Could you check a few things on this model? Use its own coordinates, in mm. A direction names the side the tool comes from. Coordinates: 2 decimals unless noted, no trailing zeros. Write each loop counter-clockwise with the first axis right and the second up, starting at its lowest first coordinate (ties: lowest second). Pieces come first, ordered by that corner, then holes.
Item 1: If I drill on probe 1 along Y at (x, z) = (-34, 4); probe 2 along Y at (x, z) = (-26.5, 8); probe 3 along Y at (x, z) = (-2, 2.5), over which ranges is the centre line in solid material (lowest first)?
Item 2: For P1, Ø6, axis at x = -31.5, y = 6, coming from the -Z side; P2, Ø1.5, axis at y = 7, z = 7, coming from the -X side; P3, Ø4, axis at y = -14, z = 7.5, coming from the -X side; P4, Ø3, axis at y = 19, z = 9, coming from the +X side, each with a flat end and sliding along its axis, tell me the tip position at first contact or that it passes through.
Item 3: I want a section at C-C on x = 41. Please give me the cut outline in (y, z), then the cut area to 3 significant figures.
Item 4: I want a section at A-A on x = 0. Please give me the cut outline in (y, z), then the cut area to 3 significant figures.
Item 5: Which directions (+Z, -Z, +X, -X, +Y, -Y) give clear straight access to the entire face, cutting with the end or side of a thin tool? Please do faces 4 (the flat face through (27, -34.127, 5)), 5 (the cylindrical face through (31.238, 9.837, 4.536)), 6 (the flat face through (-34.192, -30.183, 1.06)).
Item 6: Thinking about a two-plate mould opening in Y: for faces 1 (the cylindrical face through (-44.68, 36.27, 5.07)), 2 (the cylindrical face through (50.87, 42.69, 5.68)), 3 (the flat face through (34.667, -30.315, 7.357)), which applies, +Y half, -Y half, draft (parallel to the pull), parting line (faces both ways), or undercut?
from build123d import *

# Parameters (mm, degrees)
SKIZZE1_R                       = 32.75
AUFSATZ_LINEAR_AUSTRAGEN1_DEPTH = 10
AUFSATZ_LINEAR_START            = -0.8
SKIZZE2_R                       = 32.75
SKIZZE2_R_2                     = 30.25
AUFSATZ_LINEAR_AUSTRAGEN2_DEPTH = 0.8
SKIZZE5_R                       = 2.25
SCHNITT_LINEAR_AUSTRAGEN1_DEPTH = 10
VERRUNDUNG1_R                   = 50
VERRUNDUNG2_R                   = 6
VERRUNDUNG3_R                   = 4
AUFSATZ_LINEAR_AUSTRAGEN3_DEPTH = 8.306468


with BuildPart() as part:
    # Skizze1 → Aufsatz-Linear austragen1 (new body)
    with BuildSketch(Plane.XY):
        with BuildLine():
            Line((-13.635878322, -34.12660725), (-33.089645956, -34.12660725))
            Line((-33.089645956, -34.12660725), (-35.325135331, -26.12660725))
            Line((-35.325135331, -26.12660725), (-25.844978112, -26.12660725))
            ThreePointArc((-25.844978112, -26.12660725), (-36.75, 0), (-25.844978112, 26.12660725))
            Line((-25.844978112, 26.12660725), (-50.235580292, 27.232429468))
            Line((-50.235580292, 27.232429468), (-52.656417654, 35.895722216))
            Line((-52.656417654, 35.895722216), (-56.424186432, 49.379190555))
            Line((-56.424186432, 49.379190555), (-49.682452262, 51.263074944))
            Line((-49.682452262, 51.263074944), (-45.294995525, 35.561969729))
            Line((-45.294995525, 35.561969729), (-13.635878322, 34.12660725))
            ThreePointArc((-13.635878322, 34.12660725), (0, 36.75), (13.635878322, 34.12660725))
            Line((13.635878322, 34.12660725), (45.294995525, 35.561969729))
            Line((45.294995525, 35.561969729), (49.682452262, 51.263074944))
            Line((49.682452262, 51.263074944), (56.424186432, 49.379190555))
            Line((56.424186432, 49.379190555), (52.656417654, 35.895722216))
            Line((52.656417654, 35.895722216), (50.235580292, 27.232429468))
            Line((50.235580292, 27.232429468), (25.844978112, 26.12660725))
            ThreePointArc((25.844978112, 26.12660725), (36.75, 0), (25.844978112, -26.12660725))
            Line((25.844978112, -26.12660725), (35.325135331, -26.12660725))
            Line((35.325135331, -26.12660725), (33.089645956, -34.12660725))
            Line((33.089645956, -34.12660725), (13.635878322, -34.12660725))
            ThreePointArc((13.635878322, -34.12660725), (0, -36.75), (-13.635878322, -34.12660725))
        make_face()
        Circle(SKIZZE1_R, mode=Mode.SUBTRACT)
    extrude(amount=AUFSATZ_LINEAR_AUSTRAGEN1_DEPTH)

    # Skizze2 → Aufsatz-Linear austragen2 (add)
    with BuildSketch(Plane.XY.offset(10).offset(AUFSATZ_LINEAR_START)):
        Circle(SKIZZE2_R)
        Circle(SKIZZE2_R_2, mode=Mode.SUBTRACT)
    extrude(amount=AUFSATZ_LINEAR_AUSTRAGEN2_DEPTH)

    # Skizze5 → Schnitt-Linear austragen1 (cut)
    with BuildSketch(Plane(origin=(32.796772797, -9.164604643, 0), x_dir=(0, 0, 1), z_dir=(-0.9631048813334842, 0.2691263412444341, 0))):
        with Locations(Location((5, 56.94978804, 0), (0, 0, 270))):
            Circle(SKIZZE5_R)
    schnitt_linear_austragen1 = extrude(amount=-SCHNITT_LINEAR_AUSTRAGEN1_DEPTH, mode=Mode.SUBTRACT)

    # Spiegeln1: Schnitt-Linear austragen1 across plane
    add(schnitt_linear_austragen1.mirror(Plane(origin=(0, 0, 0), x_dir=(0, 0, 1), z_dir=(1, 0, 0))), mode=Mode.SUBTRACT)

    # Verrundung1
    verrundung1_edges = [part.edges().sort_by_distance(p)[0] for p in [
        (13.635878322, 34.12660725, 5),
        (13.635878322, -34.12660725, 5),
        (-13.635878322, -34.12660725, 5),
        (-13.635878322, 34.12660725, 5),
    ]]
    fillet(verrundung1_edges, radius=VERRUNDUNG1_R)

    # Verrundung2
    # the kernel refuses this fillet: 6 mm, written as the material it adds along each edge
    with BuildSketch(Plane(origin=(-25.844978112, -26.12660725, 0), x_dir=(-1, 0, 0), z_dir=(0, 0, 1))) as verrundung2_piece_1:
        with BuildLine():
            CenterArc((11.651069987, -5.593490659), VERRUNDUNG2_R, 111.211936516, 97.493506366)
            Line((6.388466745, -8.475331584), (6.283214681, -8.532968403))
            ThreePointArc((6.283214681, -8.532968403), (3.405977683, -4.078058883), (-0.084391765, -0.085311371))
            Line((-0.084391765, -0.085311371), (0, 0.12))
            ThreePointArc((0, 0.12), (4.74007861, 0.12), (9.436738964, 0.111869813))
            Line((9.436738964, 0.111869813), (9.48015722, 0))
        make_face()
    extrude(amount=10)
    with BuildSketch(Plane(origin=(25.844978112, -26.12660725, 0), x_dir=(1, 0, 0), z_dir=(0, 0, 1))) as verrundung2_piece_2:
        with BuildLine():
            CenterArc((11.651069987, 5.593490659), VERRUNDUNG2_R, 151.294557118, 97.493506366)
            Line((6.388466745, 8.475331584), (6.283214681, 8.532968403))
            ThreePointArc((6.283214681, 8.532968403), (3.405977683, 4.078058883), (-0.084391765, 0.085311371))
            Line((-0.084391765, 0.085311371), (0, -0.12))
            ThreePointArc((0, -0.12), (4.74007861, -0.12), (9.436738964, -0.111869813))
            Line((9.436738964, -0.111869813), (9.48015722, 0))
        make_face()
    extrude(amount=10)
    with BuildSketch(Plane(origin=(25.844978112, 26.12660725, 0), x_dir=(0.603126946859045, -0.7976452130944475, 0), z_dir=(0, 0, 1))) as verrundung2_piece_3:
        with BuildLine():
            CenterArc((11.361383868, 5.938413704), VERRUNDUNG2_R, 145.501722428, 116.281978681)
            Line((6.416524574, 9.336702474), (6.317627388, 9.40466825))
            Line((6.317627388, 9.40466825), (-0.098897186, 0.067965775))
            Line((-0.098897186, 0.067965775), (0.017149259, -0.118768274))
            ThreePointArc((0.017149259, -0.118768274), (5.251960467, 0.257216064), (10.486771676, -0.118768274))
            Line((10.486771676, -0.118768274), (10.503920934, 0))
        make_face()
    extrude(amount=10)
    with BuildSketch(Plane(origin=(-25.844978112, 26.12660725, 0), x_dir=(-0.6031269468590452, -0.7976452130944475, 0), z_dir=(0, 0, 1))) as verrundung2_piece_4:
        with BuildLine():
            CenterArc((11.361383868, -5.938413704), VERRUNDUNG2_R, 98.216298891, 116.281978681)
            Line((6.416524574, -9.336702474), (6.317627388, -9.40466825))
            Line((6.317627388, -9.40466825), (-0.098897186, -0.067965775))
            Line((-0.098897186, -0.067965775), (0.017149259, 0.118768274))
            ThreePointArc((0.017149259, 0.118768274), (5.251960467, -0.257216064), (10.486771676, 0.118768274))
            Line((10.486771676, 0.118768274), (10.503920934, 0))
        make_face()
    extrude(amount=10)

    # Verrundung3
    verrundung3_edges = [part.edges().sort_by_distance(p)[0] for p in [
        (45.294995525, 35.561969729, 5),
        (-45.294995525, 35.561969729, 5),
    ]]
    fillet(verrundung3_edges, radius=VERRUNDUNG3_R)

    # Skizze6 → Aufsatz-Linear austragen3 (add)
    with BuildSketch(Plane(origin=(6.448861011, -23.078118218, 0), x_dir=(0, 0, -1), z_dir=(-0.26912634124443396, 0.9631048813334842, 0))):
        Polygon((-7.85, 41.05316849), (-6.85, 42.05316849), (-3.15, 42.05316849), (-2.15, 41.05316849), align=None)
    aufsatz_linear_austragen3 = extrude(amount=AUFSATZ_LINEAR_AUSTRAGEN3_DEPTH)

    # Spiegeln2: Aufsatz-Linear austragen3 across plane
    add(aufsatz_linear_austragen3.mirror(Plane(origin=(0, 0, 0), x_dir=(0, 0, 1), z_dir=(1, 0, 0))))


solid = part.part
Response values:
1. probe 1: y = -34.38 to -25.41, -13.95 to 13.95, 25.57 to 35.05
1. probe 2: y = -34.13 to -19.24, 19.24 to 34.71
1. probe 3: y = -36.7 to -32.69, 32.69 to 36.7
2. P1: stops at z = 0
2. P2: stops at x = -36.21
2. P3: stops at x = -34.74
2. P4: stops at x = 32.32
3. outline: (26.81, 0) - (35.37, 0) - (35.37, 10) - (26.81, 10) - close
3. area: 85.5 mm2
4. outline: (-36.75, 0) - (-32.75, 0) - (-32.75, 9.2) - (-30.25, 9.2) - (-30.25, 10) - (-36.75, 10) - close; (30.25, 9.2) - (32.75, 9.2) - (32.75, 0) - (36.75, 0) - (36.75, 10) - (30.25, 10) - close
4. area: 84.0 mm2
5. face 4: +Z, -Z, -Y
5. face 5: -Z
5. face 6: -Z, -X, -Y
6. face 1: +Y half
6. face 2: undercut
6. face 3: -Y half
